```python
from build123d import *

# Parameters (mm, degrees)
SKETCH1_R           = 1.5625
BOSS_EXTRUDE1_DEPTH = 4.7625
FILLET1_R           = 0.5
SKETCH2_R           = 1.5
CUT_EXTRUDE1_DEPTH  = 31.457862798


with BuildPart() as part:
    # Sketch1 → Boss-Extrude1 (new body)
    with BuildSketch(Plane(origin=(0, 0, 0), x_dir=(1, 0, 0), z_dir=(0, 1, 0))):
        with BuildLine():
            Line((-1.65, 0), (1.65, 0))
            Line((1.65, 0), (1.65, -5))
            Line((1.65, -5), (2.65, -5))
            Line((2.65, -5), (2.65, 1.9))
            Line((2.65, 1.9), (1.9, 1.9))
            Line((1.9, 1.9), (1.9, 3.05))
            Line((1.9, 3.05), (2.75, 3.9))
            Line((2.75, 3.9), (4.15, 3.9))
            Line((4.15, 3.9), (4.15, -8))
            ThreePointArc((4.15, -8), (3.271320344, -10.121320344), (1.15, -11))
            Line((1.15, -11), (-24, -11))
            ThreePointArc((-24, -11), (-28, -7), (-24, -3))
            Line((-24, -3), (-5.15, -3))
            Line((-5.15, -3), (-5.15, -5))
            Line((-5.15, -5), (-4.15, -5))
            Line((-4.15, -5), (-4.15, 3.9))
            Line((-4.15, 3.9), (-2.75, 3.9))
            Line((-2.75, 3.9), (-1.9, 3.05))
            Line((-1.9, 3.05), (-1.9, 1.9))
            Line((-1.9, 1.9), (-2.65, 1.9))
            Line((-2.65, 1.9), (-2.65, -5))
            Line((-2.65, -5), (-1.65, -5))
            Line((-1.65, -5), (-1.65, 0))
        make_face()
        with Locations(Location((-24, -7, 0), (0, 0, 90))):
            Circle(SKETCH1_R, mode=Mode.SUBTRACT)
        with Locations(Location((-9, -7, 0), (0, 0, 90))):
            Circle(SKETCH1_R, mode=Mode.SUBTRACT)
    extrude(amount=BOSS_EXTRUDE1_DEPTH)

    # Fillet1
    fillet1_edges = [part.edges().sort_by_distance(p)[0] for p in [
        (-2.65, 2.38125, 5),
        (-1.65, 2.38125, 5),
        (2.65, 2.38125, 5),
        (1.65, 2.38125, 5),
        (-5.15, 2.38125, 5),
        (-4.15, 2.38125, 5),
    ]]
    fillet(fillet1_edges, radius=FILLET1_R - 0.0001)  # a hair under: the kernel refuses the full size

    # Sketch2 → Cut-Extrude1 (cut, through all)
    with BuildSketch(Plane(origin=(0, 4.7625, 0), x_dir=(1, 0, 0), z_dir=(0, 1, 0))):
        with Locations(Location((0, -7.75, 0), (0, 0, 270))):
            Circle(SKETCH2_R)
    extrude(amount=-CUT_EXTRUDE1_DEPTH, mode=Mode.SUBTRACT)


solid = part.part
```
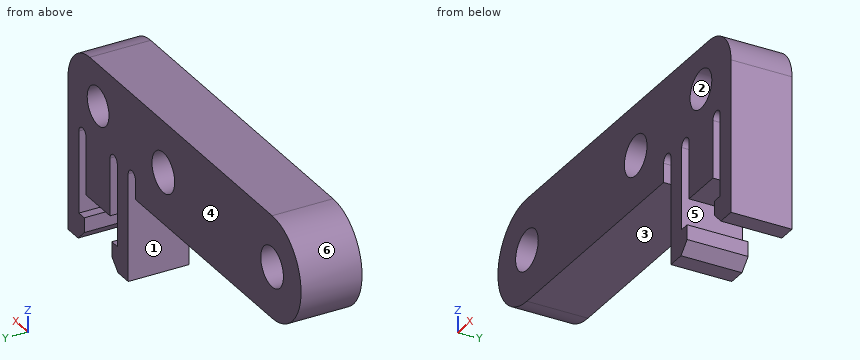
CAD build for the part. Positions are in the model's coordinates, mm. Face numbers are marked on the shaded views. A direction names the side the tool comes from. Round coordinates to 2 decimals unless told otherwise and drop trailing zeros. Write each loop counter-clockwise with the first axis right and the second up, starting at its lowest first coordinate (ties: lowest second). Pieces come first, ordered by that corner, then holes. Notation, with made-up numbers: (1.5, 62.5) - (35.5, 62.5) arc R15 cw to (35.5, 69.5) - close; hole circle Ø10 at (77, 15.5). An arc over 180 degrees is marked (long way). Write item = value, one per line. Start each with the question number.
Q1. Band-saw the part on B-B (y = 2.3). Count the separate pieces of the cut face and the enclosed holes in it, then the cut area to 3 significant figures.
Q2. Band-saw the part on C-C (z = 5.75). Give the cut face in (x, y).
Q3. Drop flat-ended pins along their axis: pin 1 (2.5 mm diameter, centred on x = 0, z = 7.75, fed in from -Y); pin 2 (4 mm diameter, centred on x = -24, z = 7, fed in from -Y); pin 3 (2.5 mm diameter, centred on y = 1.5, z = 2.5, fed in from -X); pin 4 (2 mm diameter, centred on y = 1.5, z = 0.5, fed in from -X). Give the stop position or say it passes through.
Q4. Band-saw the part on D-D (x = -17). Give the cut face in (y, z).
Q5. Mould opens along Z. For the marked faces 4, 5 and 6 say: pulls with the +Z half, pulls with the -Z half, needs draft (parallel to the pull), parting line crosses it, or undercut.
Q6. Which spindle directions (+Z, -Z, +X, -X, +Y, -Y) get a long thin tool onto all of the face, cutting with end or side? Do the marked faces 1, 2 and 3. Say none if no direction does.
Q7. Probe L1, parallel to X at y = 3.45, z = 0.25; L2, parallel to X at y = 3, z = -1.25; L3, parallel to Z at x = -24, y = 1.7. List the from-to ranges inside material, lowest first. Write a range as from..to.
Q8. Band-saw the part on A-A (x = -9). Give the cut face in (y, z).
Answers below:
q1.separate_pieces = 1
q1.enclosed_holes = 3
q1.area = 253 mm2
q2.outline = (-27.8, 0) - (-24.94, 0) - (-24.94, 4.76) - (-27.8, 4.76) - close; (-23.06, 0) - (-9.94, 0) - (-9.94, 4.76) - (-23.06, 4.76) - close; (-8.06, 0) - (4.15, 0) - (4.15, 4.76) - (-8.06, 4.76) - close
q3.pin_1 = through
q3.pin_2 = 0
q3.pin_3 = -26.33
q3.pin_4 = -4.15
q4.outline = (0, 3) - (4.76, 3) - (4.76, 11) - (0, 11) - close
q5.face_4 = needs draft
q5.face_5 = undercut
q5.face_6 = parting line crosses it
q6.face_1 = -Z, +Y, -Y
q6.face_2 = +Y, -Y
q6.face_3 = -Z, -X, +Y, -Y
q7.L1 = -4.15..-2.65, -1.65..1.65, 2.65..4.15
q7.L2 = -4.15..-2.65, 2.65..4.15
q7.L3 = 3..5.44, 8.56..11
q8.outline = (0, 3) - (4.76, 3) - (4.76, 5.44) - (0, 5.44) - close; (0, 8.56) - (4.76, 8.56) - (4.76, 11) - (0, 11) - close
